from build123d import *

# Parameters (mm, degrees)
F1_DEPTH = 10
F2_W     = 4.5
F2_H     = 4.5
F3_DEPTH = 4.5
F4_W     = 4.5
F4_H     = 4.5
F5_DEPTH = 1.5


with BuildPart() as f1:
    # F0 (on Front) → F1 (new body)
    with BuildSketch(Plane.XZ):
        Polygon((6.8, 0), (0, 0), (0, -49.2), (21.014519, 0), (13.674519, 0), (6.8, -18.95), align=None)
    extrude(amount=F1_DEPTH)

    # F2 (on face) → F3 (join)
    with BuildSketch(Plane.XY):
        with Locations((3.4, -5)):
            Rectangle(F2_W, F2_H)
    extrude(amount=F3_DEPTH)

    # F4 (on face) → F5 (join)
    with BuildSketch(Plane.XY):
        with Locations((17.344519, -5)):
            Rectangle(F4_W, F4_H)
    extrude(amount=F5_DEPTH)


solid = f1.part
Geometry check sheet. Reference: the model listing, model coordinates, mm. A direction names the side the tool comes from. Coordinates: 2 decimals unless noted, no trailing zeros. Write each loop counter-clockwise with the first axis right and the second up, starting at its lowest first coordinate (ties: lowest second). Pieces come first, ordered by that corner, then holes. Notation, with made-up numbers: (52, 27.25) -> (91, 27.25) arc R31 ccw to (91, 57.25) -> close; hole circle Ø9 at (13, 83.25). An arc over 180 degrees is marked (long way). One line per question, with ' | ' between items.
1. Thickness scan on probe 1 along X at (y, z) = (-7, -36); probe 2 along X at (y, z) = (-5, -16.5); probe 3 along X at (y, z) = (-6, -1.5). Record the ranges inside material, lowest first. Write a range as from..to.
Answers:
probe 1: x = 0..5.64 | probe 2: x = 0..6.8, 7.69..13.97 | probe 3: x = 0..6.8, 13.13..20.37
2. Cross-section at D-D on z = -28.5. Record the cut outline in (x, y).
Answers:
outline: (0, -10) -> (8.84, -10) -> (8.84, 0) -> (0, 0) -> close
3. Cross-section at C-C on x = 4.5. Record the cut outline in (y, z), and give its area (3 significant figures).
Answers:
outline: (-10, -38.66) -> (0, -38.66) -> (0, 0) -> (-2.75, 0) -> (-2.75, 4.5) -> (-7.25, 4.5) -> (-7.25, 0) -> (-10, 0) -> close | area: 407 mm²
4. Depth check by flat-ended pin: pin 1 Ø2 at (y, z) = (-6, -37.5) entering from +X; pin 2 Ø0.8 at (x, z) = (17, 0.5) entering from +Y; pin 3 Ø1.3 at (y, z) = (-5.5, 2) entering from +X. Enter the tip coordinate at first touch or a pass-through.
Answers:
pin 1: stops at x = 5.42 | pin 2: stops at y = -2.75 | pin 3: stops at x = 19.59
5. Draft check along X on faces 1 (the flat face through (10.3, -4.9, -9.3)), 2 (the flat face through (10.36, -4.93, -24.94)), 3 (the flat face through (3, -2.75, 2)). Enter one of: +X half, -X half, draft (parallel to the pull), parting line (faces both ways), or undercut.
Answers:
face 1: undercut | face 2: +X half | face 3: draft
6. Cross-section at B-B on y = -6.75. Record the cut outline in (x, z).
Answers:
outline: (0, -49.2) -> (21.01, 0) -> (19.59, 0) -> (19.59, 1.5) -> (15.09, 1.5) -> (15.09, 0) -> (13.67, 0) -> (6.8, -18.95) -> (6.8, 0) -> (5.65, 0) -> (5.65, 4.5) -> (1.15, 4.5) -> (1.15, 0) -> (0, 0) -> close
7. Cross-section at A-A on z = -13.5. Record the cut outline in (x, y), and give its area (3 significant figures).
Answers:
outline: (0, -10) -> (6.8, -10) -> (6.8, 0) -> (0, 0) -> close; (8.78, -10) -> (15.25, -10) -> (15.25, 0) -> (8.78, 0) -> close | area: 133 mm²
8. Set-up check for faces 4 (the flat face through (17, -2.75, 1)), 5 (the flat face through (5.65, -5, 2)), 6 (the flat face through (1.15, -5, 2)), 7 (the flat face through (19.595, -5, 1)): record each of +Z, -Z, +X, -X, +Y, -Y from which the full face is reachable in a straight line by a thin tool's end or side.
Answers:
face 4: +Z, +X, -X, +Y | face 5: +Z, +Y, -Y | face 6: +Z, -X, +Y, -Y | face 7: +Z, +X, +Y, -Y
